Source: CAD feature listing. Evaluate the final solid. Frame: model axes, mm. A direction names the side the tool comes from. Give positions to 0.01 mm unless a question says otherwise; leave off trailing zeros. Write each loop counter-clockwise with the first axis right and the second up, starting at its lowest first coordinate (ties: lowest second). Pieces come first, ordered by that corner, then holes. Notation, with made-up numbers: M 4,69.25 L 45,69.25 A26 cw 45,98.25 Z; hole C 2,49.5 d5. An arc over 180 degrees is marked long. Return JSON: item names as keys, results as strings.
Autodesk Inventor part; units mm, degrees
ref_plane "YZ Plane" through (0, 0, 0) normal (1, 0, 0) x (0, 1, 0)
ref_plane "XZ Plane" through (0, 0, 0) normal (0, 1, 0) x (-1, 0, 0)
ref_plane "XY Plane" through (0, 0, 0) normal (0, 0, 1) x (1, 0, 0)
sketch "Sketch1" plane through (0, 0, 0) normal (0, 1, 0) x (-1, 0, 0)
  line L0 (0, 0) -> (105, 0)
  line L1 (105, 0) -> (105, -50)
  line L2 (105, -50) -> (0, -50)
  line L3 (0, -50) -> (0, 0)
  line L4 (0, 0) -> (0, -16.6667)
  line L5 (0, -16.6667) -> (11, -16.6667)
  dimension "d0" = 105
  dimension "d1" = 50
  dimension "d2" = 16.6667
  dimension "d3" = 11
extrude "Extrusion1" add sketch "Sketch1" along normal blind 6
sketch "Sketch3" plane through (0, 6, 0) normal (0, 1, 0) x (1, 0, 0)
  circle A0 centre (-20, 12.5) radius 2.75
  line L0 (0, 0) -> (0, 50)
  line L1 (-105, 0) -> (0, 0)
  circle A1 centre (-20, 37.5) radius 2.75
  dimension "d21" = 5.5
  dimension "d22" = 20
  dimension "d23" = 12.5
  dimension "d26" = 25
extrude "Extrusion3" cut sketch "Sketch3" against normal through all
sketch "Sketch4" plane through (0, 6, 0) normal (0, 1, 0) x (1, 0, 0)
  circle A0 centre (-20, 12.5) radius 2.75
  line L0 (-20, 12.5) -> (-78, 12.5)
  line L1 (-78, 12.5) -> (-88, 12.5) construction
  line L2 (-78, 15.25) -> (-88, 15.25)
  line L3 (-88, 9.75) -> (-78, 9.75)
  arc A1 (-78, 9.75) -> (-78, 15.25) centre (-78, 12.5) ccw
  arc A2 (-88, 15.25) -> (-88, 9.75) centre (-88, 12.5) ccw
  point P0 (0, 0)
  point P1 (-83, 12.5)
  dimension "d33" = 58
  dimension "d34" = 10
  dimension "d35" = 5.5
extrude "Extrusion4" cut sketch "Sketch4" against normal through all contours A1 L3 A2 L2
pattern_linear "Rectangular Pattern2" count 2 spacing 25 along (0, 0, -1) of "Extrusion4"
sketch "Sketch5" plane through (0, 0, -50) normal (0, 0, -1) x (-1, 0, 0)
  line L0 (105, 0) -> (105, 6)
  line L1 (105, 0) -> (0, 0)
  line L2 (105, 6) -> (75, 6)
  line L3 (75, 6) -> (75, 0)
  line L4 (75, 0) -> (105, 0)
  line L5 (105, 0) -> (105, 6)
  dimension "d45" = 30
extrude "Extrusion5" add sketch "Sketch5" along normal blind 25
sketch "Sketch6" plane through (0, 6, 0) normal (0, 1, 0) x (1, 0, 0)
  line L0 (-83, 60.5) -> (-83, 70.5) construction
  line L1 (-80.25, 60.5) -> (-80.25, 70.5)
  line L2 (-85.75, 70.5) -> (-85.75, 60.5)
  arc A0 (-85.75, 60.5) -> (-80.25, 60.5) centre (-83, 60.5) ccw
  arc A1 (-80.25, 70.5) -> (-85.75, 70.5) centre (-83, 70.5) ccw
  line L3 (-75, 50) -> (-75, 75)
  arc A2 (-88, 40.25) -> (-88, 34.75) centre (-88, 37.5) ccw
  point P0 (0, 0)
  point P1 (-83, 65.5)
  dimension "d48" = 10
  dimension "d49" = 5.5
  dimension "d50" = 8
  dimension "d51" = 28
extrude "Extrusion6" cut sketch "Sketch6" against normal through all
fillet "Fillet2" radius 5 6 edges at (-105, 3, 0) (0, 3, 0) (-75, 3, -75) (-105, 3, -75) (0, 3, -50) (-75, 3, -50)
sketch "Sketch7" plane through (0, 6, 0) normal (0, 1, 0) x (1, 0, 0)
  circle A0 centre (-20, 12.5) radius 2.75
  line L0 (-20, 12.5) -> (-42, 12.5)
  line L1 (-42, 12.5) -> (-62, 12.5)
  circle A1 centre (-62, 12.5) radius 2.75
  circle A2 centre (-42, 12.5) radius 2.75
  line L2 (0, 5) -> (0, 45)
  line L3 (0, 0) -> (0, 45)
  circle A3 centre (-42, 37.5) radius 2.75
  circle A4 centre (-62, 37.5) radius 2.75
  dimension "d55" = 22
  dimension "d56" = 20
  dimension "d57" = 5.5
  dimension "d58" = 5.5
  dimension "d61" = 25
extrude "Extrusion7" cut sketch "Sketch7" against normal through all contours A1 | A2 L1 L0 | L0 L1 A2 | A3 | A4
sketch "Sketch9" plane through (0, 6, 0) normal (0, 1, 0) x (1, 0, 0)
  point P0 (0, 0)
sketch "Sketch10" plane through (0, 6, 0) normal (0, 1, 0) x (1, 0, 0)
  circle A0 centre (-100, 70) radius 2.75
  line L0 (-100, 75) -> (-80, 75)
  line L1 (-105, 5) -> (-105, 70)
  circle A1 centre (-100, 5) radius 2.75
  line L2 (-100, 0) -> (-5, 0)
  circle A2 centre (-5, 45) radius 2.75
  line L3 (-5, 50) -> (-70, 50)
  line L4 (0, 5) -> (0, 45)
  circle A3 centre (-5, 5) radius 2.75
  point P0 (0, 0)
  dimension "d70" = 5.5
  dimension "d71" = 5
  dimension "d72" = 5
  dimension "d73" = 5.5
  dimension "d74" = 5
  dimension "d75" = 5
  dimension "d76" = 5.5
  dimension "d77" = 5
  dimension "d78" = 5
  dimension "d79" = 5.5
  dimension "d80" = 5
  dimension "d81" = 5
extrude "Extrusion9" cut sketch "Sketch10" against normal through all
properties part number "X_Carriage_Plate"
1) Contact query for flat-ended pins moving along their axis: pin 1 Ø3 at (x, y) = (-43.5, 3) entering from -Z; pin 2 Ø4.5 at (x, z) = (-5, -45) entering from -Y; pin 3 Ø1.8 at (y, z) = (3, -65.5) entering from +X. Output: stop coordinate, or through.
Numbers:
{"pin 1": "stops at z = -50", "pin 2": "passes through", "pin 3": "stops at x = -75"}
2) Cut plane A-A, the plane z = -12.5. Return the cut outline in (x, y), then the cut area to 3 significant figures.
Numbers:
{"outline": "M -105,0 L -90.75,0 L -90.75,6 L -105,6 Z; M -75.25,0 L -64.75,0 L -64.75,6 L -75.25,6 Z; M -59.25,0 L -44.75,0 L -44.75,6 L -59.25,6 Z; M -39.25,0 L -22.75,0 L -22.75,6 L -39.25,6 Z; M -17.25,0 L 0,0 L 0,6 L -17.25,6 Z", "area": "438 mm²"}
3) Draft query along X for faces 1 (the face through (-75.25, 3.04, -37.44)), 2 (the face through (-53, 0, -29)), 3 (the face through (0, 3, -25)). Return one class per face: released by +X, released by -X, zero draft, split by the parting line, or undercut.
Numbers:
{"face 1": "undercut", "face 2": "zero draft", "face 3": "released by +X"}
4) Line query: line 1 (X direction, y = 3, z = -37.5); line 2 (X direction, y = 3.85, z = -70); line 3 (X direction, y = 2, z = -5). Output: solid intervals per line, ascending. Write a range as [from, to].
Numbers:
{"line 1": "x = [-105, -90.75], [-75.25, -64.75], [-59.25, -44.75], [-39.25, -22.75], [-17.25, 0]", "line 2": "x = [-105, -102.75], [-97.25, -85.75], [-80.25, -75]", "line 3": "x = [-105, -102.75], [-97.25, -7.75], [-2.25, 0]"}
5) Cut plane B-B, the plane y = 4.9. Give the number of separate pieces and of enclosed holes in the cut face, then the cut area to 3 significant figures.
Numbers:
{"separate pieces": "1", "enclosed holes": "13", "area": "5,500 mm²"}
6) Set-up query: faces 4 (the face through (-103, 3, -74)), 5 (the face through (-75.25, 3.04, -12.44)), 6 (the face through (-75, 3, -62)). Return all of +Z, -Z, +X, -X, +Y, -Y with unobstructed straight access to the full face (end or side cutting, diameter ignored); none if empty.
Numbers:
{"face 4": "-Z, -X, +Y, -Y", "face 5": "+Y, -Y", "face 6": "-Z, +X, +Y, -Y"}
7) Cut plane C-C, the plane x = -83. Return the cut outline in (y, z), then the cut area to 3 significant figures.
Numbers:
{"outline": "M 0,-75 L 6,-75 L 6,-73.25 L 0,-73.25 Z; M 0,-57.75 L 6,-57.75 L 6,-40.25 L 0,-40.25 Z; M 0,-34.75 L 6,-34.75 L 6,-15.25 L 0,-15.25 Z; M 0,-9.75 L 6,-9.75 L 6,0 L 0,0 Z", "area": "291 mm²"}
8) Cut plane D-D, the plane x = -20. Return the cut outline in (y, z).
Numbers:
{"outline": "M 0,-50 L 6,-50 L 6,-40.25 L 0,-40.25 Z; M 0,-34.75 L 6,-34.75 L 6,-15.25 L 0,-15.25 Z; M 0,-9.75 L 6,-9.75 L 6,0 L 0,0 Z"}
